```python
from build123d import *

# Parameters (mm, degrees)
F0_R     = 9.875
F0_R_2   = 4.875
F1_DEPTH = 8
F0_R_3   = 17.0942544143
F2_DEPTH = 5
F3_R     = 4.8718969607
F4_DEPTH = 25


with BuildPart() as f1:
    # F0 (on Top) → F1 (new body)
    with BuildSketch(Plane.XY):
        Circle(F0_R)
        Circle(F0_R_2, mode=Mode.SUBTRACT)
        Circle(F0_R_2)
    extrude(amount=F1_DEPTH)

    # F0 (on Top) → F2 (join)
    with BuildSketch(Plane.XY):
        Circle(F0_R_3)
        Circle(F0_R, mode=Mode.SUBTRACT)
    extrude(amount=F2_DEPTH)

    # F3 (on face) → F4 (cut)
    with BuildSketch(Plane.XY.offset(8)):
        Circle(F3_R)
    extrude(amount=-F4_DEPTH, mode=Mode.SUBTRACT)


solid = f1.part
```
For this review, take the finished solid that the model builds, in its own axes (mm). Give positions to 0.01 mm unless a question says otherwise; leave off trailing zeros. Loops run counter-clockwise (first coordinate to the right, second up) from the corner with the lowest first, then second, coordinate; pieces in that order, holes last. Notation, with made-up numbers: M 28,-38.5 L 49,-38.5 A14 cw 49,-18.5 Z; hole C 66,-35.5 d2. An arc over 180 degrees is marked long. One line per item, written item: value. Start each with the question number.
Q1. Add section D-D (x = -7). Give the boundary of the cut face in (y, z).
Q2. Clearance check with flat-ended pins moving along their axes: pin 1 Ø1 at (x, z) = (2, 1) entering from -Y; pin 2 Ø2 at (x, z) = (-13, 5) entering from +Y. State where each tip first meets the part, or that it passes through.
Q3. Add section A-A (y = 0). Give the boundary of the cut face in (x, z) (3 decimals), and give its area (3 significant figures).
Q4. Draft analysis for pull direction Y (two halves, no side actions). For faces 1 (the face through (4.65, 1.46, 4.06)), 2 (the face through (-7.28, 6.67, 6.48)), 3 (the face through (7.4, -7.4, 5)), state which applies: released by +Y, released by -Y, zero draft, split by the parting line, or undercut.
Q5. For L1, parallel to Y at x = 0, z = 6.25 (3 decimals); L2, parallel to Z at x = -12, y = 6; L3, parallel to Y at x = 0, z = 3.5, list the stretches that pass through material, from the lowest coordinate up.
Q6. Add section C-C (z = 0.75). Give the boundary of the cut face in (x, y).
Reply:
1. outline: M -15.6,0 L 15.6,0 L 15.6,5 L 6.97,5 L 6.97,8 L -6.97,8 L -6.97,5 L -15.6,5 Z
2. pin 1: y = -17.03
2. pin 2: y = 12.17
3. outline: M -17.094,0 L -4.872,0 L -4.872,8 L -9.875,8 L -9.875,5 L -17.094,5 Z; M 4.872,0 L 17.094,0 L 17.094,5 L 9.875,5 L 9.875,8 L 4.872,8 Z
3. area: 152 mm²
4. face 1: undercut
4. face 2: split by the parting line
4. face 3: zero draft
5. L1: -9.875 to -4.872, 4.872 to 9.875
5. L2: 0 to 5
5. L3: -17.09 to -4.87, 4.87 to 17.09
6. outline: C 0,0 d34.19; hole C 0,0 d9.74
